from build123d import *

# Parameters (mm, degrees)
SKETCH2_W           = 50.8
SKETCH2_H           = 24.9047
SKETCH2_W_2         = 7.62
SKETCH2_H_2         = 257.175
SKETCH2_W_3         = 21.971
SKETCH2_H_3         = 16.51
SKETCH2_W_4         = 21.7424
BOSS_EXTRUDE1_DEPTH = 43.942
SKETCH2_6_W         = 7.62
SKETCH2_6_H         = 257.175
SKETCH2_6_W_2       = 21.971
SKETCH2_6_H_2       = 16.51
SKETCH2_6_W_3       = 21.7424
SKETCH2_6_W_4       = 50.8
SKETCH2_6_H_3       = 24.9047
BOSS_EXTRUDE3_DEPTH = 21.844


with BuildPart() as part:
    # Sketch2 → Boss-Extrude1 (new body)
    with BuildSketch(Plane.XY):
        with Locations((0, 409.82265)):
            Rectangle(SKETCH2_W, SKETCH2_H)
        Polygon((-25.4, 397.3703), (-25.4, 384.175), (92.329, 384.175), (92.329, 422.275), (25.4, 422.275), (25.4, 397.3703), align=None)
        with Locations((-29.21, 255.5875)):
            Rectangle(SKETCH2_W_2, SKETCH2_H_2)
        Polygon((92.329, 384.175), (-25.4, 384.175), (-25.4, 316.865), (-3.429, 316.865), (-3.429, 300.355), (-25.4, 300.355), (-25.4, 201.93), (-3.6576, 201.93), (-3.6576, 185.42), (-25.4, 185.42), (-25.4, 127), (92.329, 127), align=None)
        with Locations((-14.4145, 308.61)):
            Rectangle(SKETCH2_W_3, SKETCH2_H_3)
        with Locations((-14.5288, 193.675)):
            Rectangle(SKETCH2_W_4, SKETCH2_H_3)
        with Locations((96.139, 255.5875)):
            Rectangle(SKETCH2_W_2, SKETCH2_H_2)
        Polygon((92.329, 113.7158), (92.329, 127), (-25.4, 127), (-25.4, 88.2904), (32.21228, 88.2904), (74.6506, 113.7158), align=None)
    extrude(amount=-BOSS_EXTRUDE1_DEPTH)

    # Sketch2_6 → Boss-Extrude3 (add)
    with BuildSketch(Plane.XY):
        with Locations((-29.21, 255.5875)):
            Rectangle(SKETCH2_6_W, SKETCH2_6_H)
        with Locations((-14.4145, 308.61)):
            Rectangle(SKETCH2_6_W_2, SKETCH2_6_H_2)
        with Locations((-14.5288, 193.675)):
            Rectangle(SKETCH2_6_W_3, SKETCH2_6_H_2)
        with Locations((0, 409.82265)):
            Rectangle(SKETCH2_6_W_4, SKETCH2_6_H_3)
    extrude(amount=BOSS_EXTRUDE3_DEPTH)


solid = part.part
Could you check a few things on this model? Use its own coordinates, in mm. A direction names the side the tool comes from. Coordinates: 2 decimals unless noted, no trailing zeros. Order: outer loops, then holes, each group sorted by start corner. A loop starts at its lowest first (then second) coordinate and runs counter-clockwise, first axis right, second up.
Q1. Suppose I cut it at C-C on y = 176. Please give me the cut outline in (x, z), and give its area (3 significant figures).
Q2. Suppose I cut it at D-D on z = -23. Please give me the cut outline in (x, y) (3 decimals), and give its area (4 significant figures).
Q3. Suppose I cut it at B-B on x = -17.5. Please give me the cut outline in (y, z) (3 decimals).
Q4. Will these pins go through, and if not, where does the flat tip stop? pin 1 (8.5 mm diameter, centred on x = -30.5, z = -7.5, fed in from -Y); pin 2 (4 mm diameter, centred on x = 81, y = 148.5, fed in from +Z); pin 3 (24 mm diameter, centred on y = 409, z = 10, fed in from +X); pin 4 (17.5 mm diameter, centred on y = 252.5, z = 6, fed in from +X).
Q5. Please list where these lines run through material, in increasing order: L1, parallel to X at y = 114.5, z = -6; L2, parallel to Y at x = 9, z = 3 (3 decimals); L3, parallel to Z at x = 73.5, y = 164.5.
Q6. Suppose I cut it at A-A on z = 13. Please give me the cut outline in (x, y) (3 decimals).
Q7. Thinking about a two-plate mould opening in Y: for faces 1 (the flat face through (96, 127, -22)), 2 (the flat face through (-25.4, 108, -22)), 3 (the flat face through (34, 422.275, -18)), 4 (the flat face through (-15, 201.93, 11)), which applies, released by +Y, released by -Y, zero draft, split by the parting line, or undercut?
Q8. Which directions (+Z, -Z, +X, -X, +Y, -Y) give clear straight access to the entire face, cutting with the end or side of a thin tool? Please do faces 5 (the flat face through (-29, 127, -12)), 6 (the flat face through (0, 397.37, 11)), 7 (the flat face through (-25.4, 250, 11)), 8 (the flat face through (92.329, 403, -22)).
Answer:
1. outline: (-33.02, -43.94) - (99.95, -43.94) - (99.95, 0) - (-25.4, 0) - (-25.4, 21.84) - (-33.02, 21.84) - close
1. area: 6,010 mm2
2. outline: (-33.02, 127) - (-25.4, 127) - (-25.4, 88.29) - (32.212, 88.29) - (74.651, 113.716) - (92.329, 113.716) - (92.329, 127) - (99.949, 127) - (99.949, 384.175) - (92.329, 384.175) - (92.329, 422.275) - (-25.4, 422.275) - (-25.4, 384.175) - (-33.02, 384.175) - close
2. area: 42,250 mm2
3. outline: (88.29, -43.942) - (422.275, -43.942) - (422.275, 21.844) - (397.37, 21.844) - (397.37, 0) - (316.865, 0) - (316.865, 21.844) - (300.355, 21.844) - (300.355, 0) - (201.93, 0) - (201.93, 21.844) - (185.42, 21.844) - (185.42, 0) - (88.29, 0) - close
4. pin 1: stops at y = 127
4. pin 2: stops at z = 0
4. pin 3: stops at x = 92.33
4. pin 4: stops at x = 99.95
5. L1: x = -25.4 to 92.33
5. L2: y = 397.37 to 422.275
5. L3: z = -43.94 to 0
6. outline: (-33.02, 127) - (-25.4, 127) - (-25.4, 185.42) - (-3.658, 185.42) - (-3.658, 201.93) - (-25.4, 201.93) - (-25.4, 300.355) - (-3.429, 300.355) - (-3.429, 316.865) - (-25.4, 316.865) - (-25.4, 384.175) - (-33.02, 384.175) - close; (-25.4, 397.37) - (25.4, 397.37) - (25.4, 422.275) - (-25.4, 422.275) - close
7. face 1: released by -Y
7. face 2: zero draft
7. face 3: released by +Y
7. face 4: undercut
8. face 5: +Z, -Z, -X, -Y
8. face 6: +Z, +X, -X
8. face 7: +Z, +X
8. face 8: +Z, -Z, +X, +Y
